Input: dimensioned drawing with shaded views. Units: mm. Origin: part minimum x, y, z. Round coordinates to 2 decimals unless told otherwise and drop trailing zeros. Order: outer loops, then holes, each group sorted by start corner. A loop starts at its lowest first (then second) coordinate and runs counter-clockwise, first axis right, second up.
Item 1: First-contact query: pin 1 (6 mm diameter, centred on x = 100, z = 20, fed in from -Y); pin 2 (3 mm diameter, centred on x = 38, z = 36, fed in from -Y). Flat tips, straight axial feed; report the tip coordinate or a pass-through.
Item 2: Cut plane B-B on y = 1.35. Output: boundary loops of the cut face in (x, z).
Item 3: Cut plane C-C on z = 60. Output: boundary loops of the cut face in (x, y).
Item 4: Cut plane A-A on x = 60. Output: boundary loops of the cut face in (y, z).
Item 5: Cut plane D-D on z = 16.5. Output: boundary loops of the cut face in (x, y).
Item 6: Line query: L1, parallel to Z at x = 100, y = 1.55; L2, parallel to X at y = 0.55, z = 58.5; L3, parallel to Z at x = 30, y = 1.8. Output: solid intervals per line, ascending.
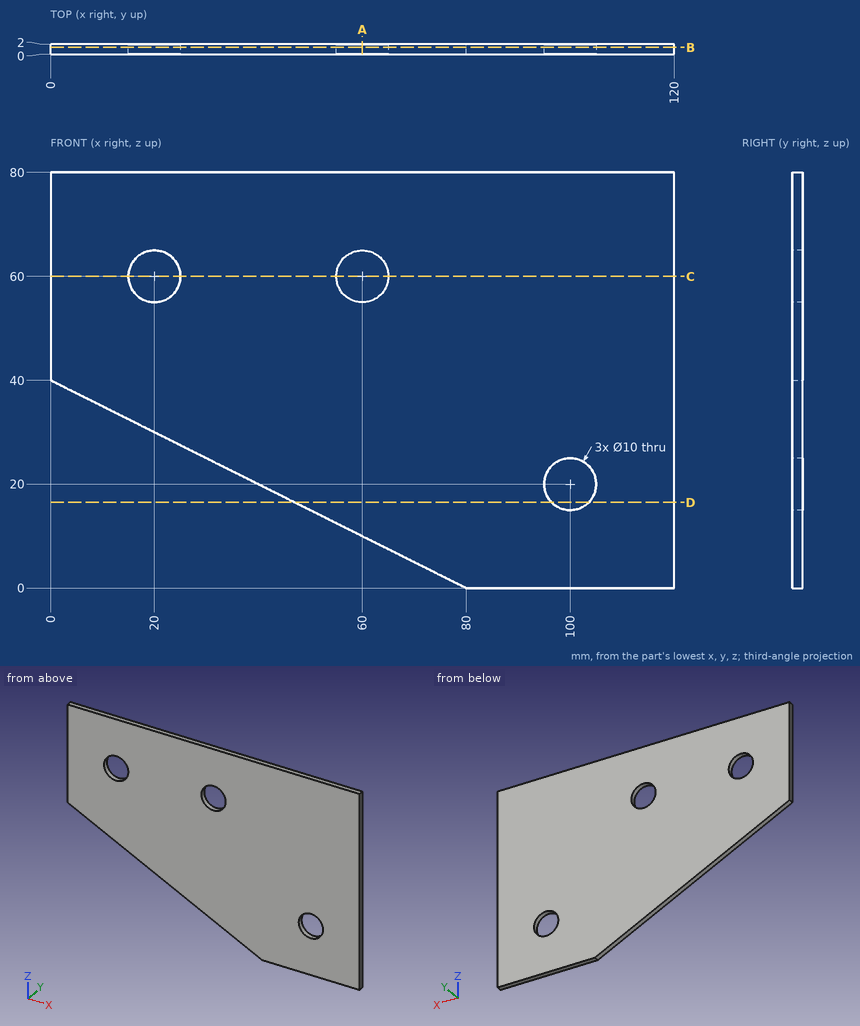
From the geometry:
1. pin 1: passes through
1. pin 2: stops at y = 0
2. outline: (0, 40) - (80, 0) - (120, 0) - (120, 80) - (0, 80) - close; hole circle Ø10 at (20, 60); hole circle Ø10 at (60, 60); hole circle Ø10 at (100, 20)
3. outline: (0, 0) - (15, 0) - (15, 2) - (0, 2) - close; (25, 0) - (55, 0) - (55, 2) - (25, 2) - close; (65, 0) - (120, 0) - (120, 2) - (65, 2) - close
4. outline: (0, 10) - (2, 10) - (2, 55) - (0, 55) - close; (0, 65) - (2, 65) - (2, 80) - (0, 80) - close
5. outline: (47, 0) - (96.43, 0) - (96.43, 2) - (47, 2) - close; (103.57, 0) - (120, 0) - (120, 2) - (103.57, 2) - close
6. L1: z = 0 to 15, 25 to 80
6. L2: x = 0 to 15.23, 24.77 to 55.23, 64.77 to 120
6. L3: z = 25 to 80
